from build123d import *

# Parameters (mm, degrees)
SKETCH3_R                = 7.874
BOSS_EXTRUDE1_DEPTH      = 14.224
BOSS_EXTRUDE1_DEPTH_BACK = 11.176
CUT_EXTRUDE1_DEPTH       = 36.052
CUT_EXTRUDE2_DEPTH       = 48.752
FILLET1_R                = 5.1435


with BuildPart() as part:
    # Sketch3 → Boss-Extrude1 (new body, two sides)
    with BuildSketch(Plane.XY) as boss_extrude1_sk:
        with BuildLine():
            Line((-23.876, 0), (23.876, 0))
            Line((23.876, 0), (23.876, 6.35))
            Line((23.876, 6.35), (12.542250985, 27.537256011))
            ThreePointArc((12.542250985, 27.537256011), (0, 35.052), (-12.542250985, 27.537256011))
            Line((-12.542250985, 27.537256011), (-23.876, 6.35))
            Line((-23.876, 6.35), (-23.876, 0))
        make_face()
        with Locations((0, 20.574)):
            Circle(SKETCH3_R, mode=Mode.SUBTRACT)
    extrude(amount=BOSS_EXTRUDE1_DEPTH)
    extrude(boss_extrude1_sk.sketch, amount=-BOSS_EXTRUDE1_DEPTH_BACK)

    # Sketch4 → Cut-Extrude1 (cut, through all)
    with BuildSketch(Plane(origin=(0, 0, 0), x_dir=(1, 0, 0), z_dir=(0, 1, 0))):
        with BuildLine():
            Line((-23.876, 3.429), (-23.876, -3.429))
            Line((-23.876, -3.429), (-19.05, -3.429))
            ThreePointArc((-19.05, -3.429), (-15.621, 0), (-19.05, 3.429))
            Line((-19.05, 3.429), (-23.876, 3.429))
        make_face()
        with BuildLine():
            Line((19.05, 3.429), (23.876, 3.429))
            Line((23.876, 3.429), (23.876, -3.429))
            Line((23.876, -3.429), (19.05, -3.429))
            ThreePointArc((19.05, -3.429), (15.621, 0), (19.05, 3.429))
        make_face()
    extrude(amount=CUT_EXTRUDE1_DEPTH, mode=Mode.SUBTRACT)

    # Sketch5 → Cut-Extrude2 (cut, through all)
    with BuildSketch(Plane.ZY.offset(23.876)):
        with BuildLine():
            Line((-11.176, 35.052), (11.176, 35.052))
            Line((11.176, 35.052), (11.176, 4.572))
            ThreePointArc((11.176, 4.572), (10.729630735, 3.494369265), (9.652, 3.048))
            Line((9.652, 3.048), (-11.176, 3.048))
            Line((-11.176, 3.048), (-11.176, 35.052))
        make_face()
        with BuildLine():
            Line((9.652, 0), (14.224, 0))
            Line((14.224, 0), (14.224, 4.572))
            ThreePointArc((14.224, 4.572), (12.884892204, 1.339107796), (9.652, 0))
        make_face()
    extrude(amount=-CUT_EXTRUDE2_DEPTH, mode=Mode.SUBTRACT)

    # Fillet1
    fillet1_edges = [part.edges().sort_by_distance(p)[0] for p in [
        (23.876, 1.524, -11.176),
        (-23.876, 1.524, -11.176),
    ]]
    fillet(fillet1_edges, radius=FILLET1_R)


solid = part.part
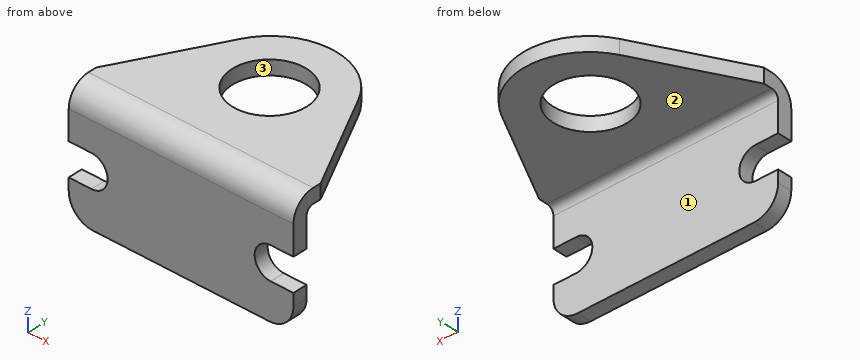
Could you check a few things on this model? Use its own coordinates, in mm. Face numbers are marked on the shaded views. Give positions to 0.01 mm unless a question says otherwise; leave off trailing zeros. Write each loop counter-clockwise with the first axis right and the second up, starting at its lowest first coordinate (ties: lowest second). Pieces come first, ordered by that corner, then holes. Notation, with made-up numbers: (54.25, 39) -> (79.25, 39) arc R30 ccw to (79.25, 74) -> close; hole circle Ø8 at (-30.75, -35.5). An arc over 180 degrees is marked (long way). Answer as a JSON object with one key per item and string values.
Q1. Suppose I cut it at B-B on y = 17.5. Write out the boundary of the cut face in (x, z).
Taken from the geometry:
{"outline": "(-17.91, 11.18) -> (-7.25, 11.18) -> (-7.25, 14.22) -> (-17.91, 14.22) -> close; (7.25, 11.18) -> (17.91, 11.18) -> (17.91, 14.22) -> (7.25, 14.22) -> close"}
Q2. Please list where these lines run through material, in increasing order: L1, parallel to Z at x = 17.5, y = 17; L2, parallel to Y at x = 0, z = 12.1; L3, parallel to Y at x = 8.5, z = 1.25.
Taken from the geometry:
{"L1": "z = 11.18 to 14.22", "L2": "y = 0.71 to 12.7, 28.45 to 35.05", "L3": "y = 0 to 3.05"}
Q3. Suppose I cut it at C-C on x = -20. Write out the boundary of the cut face in (y, z).
Taken from the geometry:
{"outline": "(0, -11.02) -> (3.05, -11.02) -> (3.05, -3.43) -> (0, -3.43) -> close; (0, 3.43) -> (3.05, 3.43) -> (3.05, 9.65) arc R1.52 cw to (4.57, 11.18) -> (13.6, 11.18) -> (13.6, 14.22) -> (4.57, 14.22) arc R4.57 ccw to (0, 9.65) -> close"}
Q4. We'd pull the mould along Y, two halves only. Please class the marked faces 1, 2 and 3: released by +Y, released by -Y, zero draft, split by the parting line, or undercut.
Taken from the geometry:
{"face 1": "released by +Y", "face 2": "zero draft", "face 3": "undercut"}
Q5. Suppose I cut it at D-D on z = 0. Write out the boundary of the cut face in (x, y).
Taken from the geometry:
{"outline": "(-15.62, 0) -> (15.62, 0) -> (15.62, 3.05) -> (-15.62, 3.05) -> close"}
Q6. Will these pins go through, and if not, where does the flat tip stop? pin 1 Ø1.5 at (x, y) = (20.5, 2.5) entering from -Z; pin 2 Ø2.5 at (x, y) = (21, 1) entering from +Z; pin 3 Ø0.9 at (x, y) = (-21, 1.5) entering from -Z.
Taken from the geometry:
{"pin 1": "stops at z = -11.07", "pin 2": "stops at z = 13.59", "pin 3": "stops at z = -10.84"}
Q7. Suppose I cut it at A-A on x = 0. Write out the boundary of the cut face in (y, z), then the cut area to 3 significant figures.
Taken from the geometry:
{"outline": "(0, -11.18) -> (3.05, -11.18) -> (3.05, 9.65) arc R1.52 cw to (4.57, 11.18) -> (12.7, 11.18) -> (12.7, 14.22) -> (4.57, 14.22) arc R4.57 ccw to (0, 9.65) -> close; (28.45, 11.18) -> (35.05, 11.18) -> (35.05, 14.22) -> (28.45, 14.22) -> close", "area": "123 mm²"}
